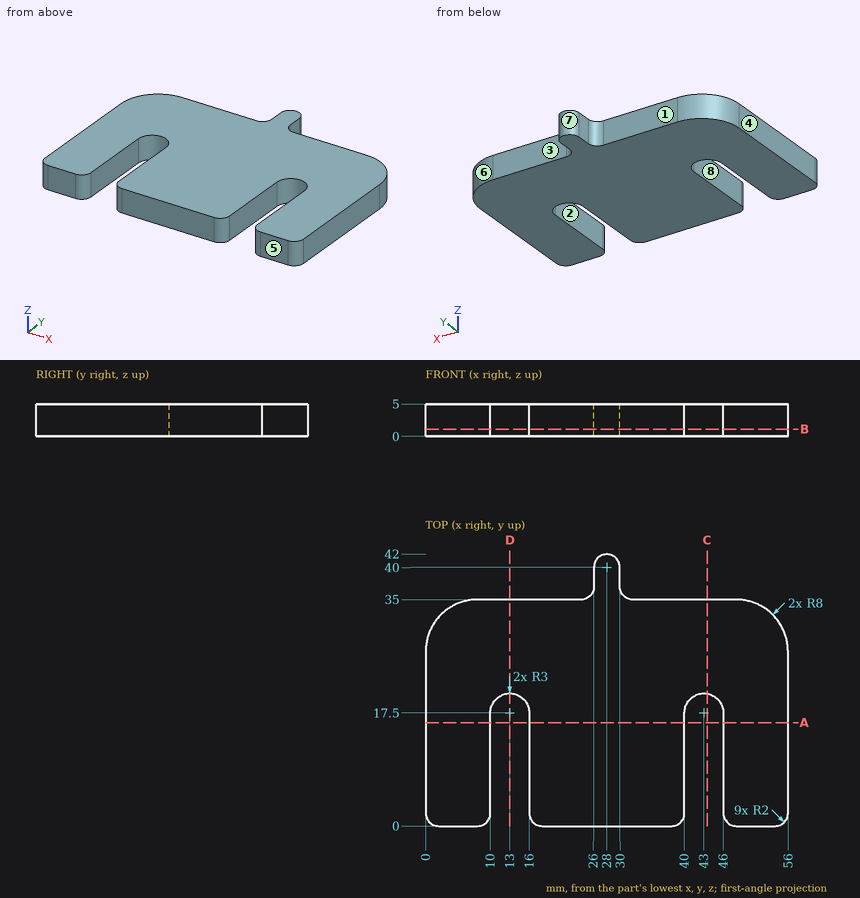
Could you check a few things on this drawing? It's one solid part, dimensions in mm from its lowest x, y, z. A direction names the side the tool comes from. Coordinates: 2 decimals unless noted, no trailing zeros. Write each loop counter-clockwise with the first axis right and the second up, starting at its lowest first coordinate (ties: lowest second). Pieces come first, ordered by that corner, then holes. Notation, with made-up numbers: (-10.5, 8) - (44.5, 8) arc R17 ccw to (44.5, 28) - close; hole circle Ø7 at (1.5, 57.5). An arc over 180 degrees is marked (long way). Put each result on its own line as item: value. Start each with the question number.
Q1. I want a section at A-A on y = 16. Write out the boundary of the cut face in (x, z).
Q2. I want a section at D-D on x = 13. Write out the boundary of the cut face in (y, z).
Q3. Please list where these lines run through material, in increasing order: L1, parallel to X at y = 9, z = 1.05; L2, parallel to X at y = 38, z = 2; L3, parallel to Y at x = 13, z = 1.2.
Q4. I want a section at C-C on x = 43.5. Write out the boundary of the cut face in (y, z), plus the area to 3 significant figures.
Q5. I'm going to push flat-ended pins straight in: P1, Ø1.5, axis at y = 38.5, z = 1.5, coming from the -X side; P2, Ø1.5, axis at x = 43, z = 3, coming from the +Y side. Where does each tip first touch, or does it pass through?
Q6. Thinking about a two-plate mould opening in X: for the marked faces 5, 6, 7 and 8, which applies, pulls with the +X half, pulls with the -X half, needs draft (parallel to the pull), parting line crosses it, or undercut?
Q7. I want a section at B-B on z = 1.1. Write out the boundary of the cut face in (x, y), plus the area to 3 significant figures.
Q8. Which directions (+Z, -Z, +X, -X, +Y, -Y) give clear straight access to the entire face, cutting with the end or side of a thin tool? Please do the marked faces 1, 2, 3 and 4.
Checks:
1. outline: (0, 0) - (10, 0) - (10, 5) - (0, 5) - close; (16, 0) - (40, 0) - (40, 5) - (16, 5) - close; (46, 0) - (56, 0) - (56, 5) - (46, 5) - close
2. outline: (20.5, 0) - (35, 0) - (35, 5) - (20.5, 5) - close
3. L1: 0 to 10, 16 to 40, 46 to 56
3. L2: 26 to 30
3. L3: 20.5 to 35
4. outline: (20.46, 0) - (35, 0) - (35, 5) - (20.46, 5) - close
4. area: 72.7 mm²
5. P1: x = 26
5. P2: y = 35
6. face 5: needs draft
6. face 6: pulls with the +X half
6. face 7: parting line crosses it
6. face 8: undercut
7. outline: (0, 2) arc R2 ccw to (2, 0) - (8, 0) arc R2 ccw to (10, 2) - (10, 17.5) arc R3 cw to (16, 17.5) - (16, 2) arc R2 ccw to (18, 0) - (38, 0) arc R2 ccw to (40, 2) - (40, 17.5) arc R3 cw to (46, 17.5) - (46, 2) arc R2 ccw to (48, 0) - (54, 0) arc R2 ccw to (56, 2) - (56, 27) arc R8 ccw to (48, 35) - (32, 35) arc R2 cw to (30, 37) - (30, 40) arc R2 ccw to (26, 40) - (26, 37) arc R2 cw to (24, 35) - (8, 35) arc R8 ccw to (0, 27) - close
7. area: 1,720 mm²
8. face 1: +Z, -Z, -X, +Y
8. face 2: +Z, -Z, -Y
8. face 3: +Z, -Z, +X, +Y
8. face 4: +Z, -Z, -X, +Y, -Y
